Here's how the part is built. I have some questions about the finished solid (model axes, mm). A direction names the side the tool comes from. Give positions to 0.01 mm unless a question says otherwise; leave off trailing zeros. Write each loop counter-clockwise with the first axis right and the second up, starting at its lowest first coordinate (ties: lowest second). Pieces come first, ordered by that corner, then holes. Notation, with made-up numbers: (-34.5, 50) -> (-26.5, 50) arc R19 ccw to (-26.5, 64) -> close; hole circle Ø7 at (43.5, -35). An arc over 180 degrees is marked (long way). Use one line per item in the form item = value.
```python
from build123d import *

# Parameters (mm, degrees)
SM_BASE_FLANGE_1_DEPTH   = 80
CUT_EXTRUDE_3_DEPTH      = 100.206854602
CUT_EXTRUDE_3_DEPTH_BACK = 100.206854602
SKETCH_6_R               = 36
SKETCH_6_R_2             = 2
FILLET_1_R               = 5
SKETCH_9_R               = 2
CUT_EXTRUDE_4_DEPTH      = 91.217792037


# Sheet-metal steps are written as plain solids
with BuildPart() as part:
    # Sketch 1 → Базовая кромка1 (new body)
    with BuildSketch(Plane.XY):
        with BuildLine():
            Line((-21.5, 29), (-21.5, 1))
            ThreePointArc((-21.5, 1), (-21.207106781, 0.292893219), (-20.5, 0))
            Line((-20.5, 0), (20.5, 0))
            ThreePointArc((20.5, 0), (21.207106781, 0.292893219), (21.5, 1))
            Line((21.5, 1), (21.5, 29))
            Line((21.5, 29), (25.5, 29))
            Line((25.5, 29), (25.5, 1))
            ThreePointArc((25.5, 1), (24.035533906, -2.535533906), (20.5, -4))
            Line((20.5, -4), (-20.5, -4))
            ThreePointArc((-20.5, -4), (-24.035533906, -2.535533906), (-25.5, 1))
            Line((-25.5, 1), (-25.5, 29))
            Line((-25.5, 29), (-21.5, 29))
        make_face()
    extrude(amount=SM_BASE_FLANGE_1_DEPTH)

    # Эскиз6 → Вырез-Вытянуть3 (cut, two sides: drawn at the far end of the back side and taken through both)
    with BuildSketch(Plane.ZY.offset(25.5).offset(-CUT_EXTRUDE_3_DEPTH_BACK)):
        with Locations((40, 52)):
            Circle(SKETCH_6_R)
        with Locations((40, 10)):
            Circle(SKETCH_6_R_2)
        with Locations((15.313019404, 18.021286236)):
            Circle(SKETCH_6_R_2)
        with Locations((64.686980596, 18.021286236)):
            Circle(SKETCH_6_R_2)
    extrude(amount=CUT_EXTRUDE_3_DEPTH + CUT_EXTRUDE_3_DEPTH_BACK, mode=Mode.SUBTRACT)

    # Скругление1
    fillet_1_edges = [part.edges().sort_by_distance(p)[0] for p in [
        (23.5, 29, 12.305235152),
        (23.5, 29, 67.694764848),
        (-23.5, 29, 12.305235152),
        (-23.5, 29, 67.694764848),
    ]]
    fillet(fillet_1_edges, radius=FILLET_1_R)

    # Эскиз9 → Вырез-Вытянуть4 (cut, through all)
    with BuildSketch(Plane.XZ.offset(4)):
        with Locations((15.5, 40)):
            Circle(SKETCH_9_R)
        with Locations((7.75, 26.576606241)):
            Circle(SKETCH_9_R)
        with Locations((-7.75, 26.576606241)):
            Circle(SKETCH_9_R)
        with Locations((-15.5, 40)):
            Circle(SKETCH_9_R)
        with Locations((-7.75, 53.423393759)):
            Circle(SKETCH_9_R)
        with Locations((7.75, 53.423393759)):
            Circle(SKETCH_9_R)
    extrude(amount=-CUT_EXTRUDE_4_DEPTH, mode=Mode.SUBTRACT)


solid = part.part
```
Q1. If I drill on line 1 along X through (y, z) = (11, 71.5); line 2 along Y through (x, z) = (-3.5, 21.5); line 3 along Z through (x, y) = (24.35, 10), over which ranges is the centre line in solid material (lowest first)? Write a range as from..to.
Result set:
line_1 = -25.5..-21.5, 21.5..25.5
line_2 = -4..0
line_3 = 0..38, 42..80
Q2. Which directions (+Z, -Z, +X, -X, +Y, -Y) give clear straight access to the entire face, cutting with the end or side of a thin tool? Please do faces 1 (the face through (7.49, -2.028, 55.406)), 2 (the face through (-23.472, 28.575, 12.067)).
Result set:
face_1 = +Y, -Y
face_2 = +X, -X, +Y
Q3. Will these pins go through, and if not, where does the flat tip stop? pin 1 Ø2.5 at (x, z) = (7.75, 26.58) entering from -Y; pin 2 Ø4.5 at (x, z) = (15.5, 40) entering from +Y.
Result set:
pin_1 = through
pin_2 = 0
Q4. If we mould it in two halves opening along Z, with no side actions, what happens to faces 3 (the face through (-23.472, 16.247, 65.61)), 4 (the face through (-2, -1, 0)), 5 (the face through (-21.5, 12, 39))? For each: +Z half, -Z half, draft (parallel to the pull), parting line (faces both ways), or undercut.
Result set:
face_3 = undercut
face_4 = -Z half
face_5 = draft
Q5. I want a section at A-A, the plane y = 7. Write out the boundary of the cut face in (x, z), and give its area (3 significant figures).
Result set:
outline = (-25.5, 0) -> (-21.5, 0) -> (-21.5, 80) -> (-25.5, 80) -> close; (21.5, 0) -> (25.5, 0) -> (25.5, 80) -> (21.5, 80) -> close
area = 640 mm2
Q6. I want a section at C-C, the plane z = 40. Write out the boundary of the cut face in (x, y).
Result set:
outline = (-25.5, 1) arc R5 ccw to (-20.5, -4) -> (-17.5, -4) -> (-17.5, 0) -> (-20.5, 0) arc R1 cw to (-21.5, 1) -> (-21.5, 8) -> (-25.5, 8) -> close; (-25.5, 12) -> (-21.5, 12) -> (-21.5, 16) -> (-25.5, 16) -> close; (-13.5, -4) -> (13.5, -4) -> (13.5, 0) -> (-13.5, 0) -> close; (17.5, -4) -> (20.5, -4) arc R5 ccw to (25.5, 1) -> (25.5, 8) -> (21.5, 8) -> (21.5, 1) arc R1 cw to (20.5, 0) -> (17.5, 0) -> close; (21.5, 12) -> (25.5, 12) -> (25.5, 16) -> (21.5, 16) -> close
Q7. I want a section at D-D, the plane x = 15.5. Write out the boundary of the cut face in (y, z).
Result set:
outline = (-4, 0) -> (0, 0) -> (0, 38) -> (-4, 38) -> close; (-4, 42) -> (0, 42) -> (0, 80) -> (-4, 80) -> close
Q8. I want a section at B-B, the plane x = 7.75. Write out the boundary of the cut face in (y, z).
Result set:
outline = (-4, 0) -> (0, 0) -> (0, 24.58) -> (-4, 24.58) -> close; (-4, 28.58) -> (0, 28.58) -> (0, 51.42) -> (-4, 51.42) -> close; (-4, 55.42) -> (0, 55.42) -> (0, 80) -> (-4, 80) -> close
